Read the model definition and answer for the solid it produces. Units are mm, in the model's axes. Give positions to 0.01 mm unless a question says otherwise; leave off trailing zeros. Order: outer loops, then holes, each group sorted by start corner. A loop starts at its lowest first (then second) coordinate and runs counter-clockwise, first axis right, second up.
Item 1: Given pin 1 Ø1 at (y, z) = (-19.5, 2) entering from +X; pin 2 Ø3 at (y, z) = (-12, 17.5) entering from +X; pin 3 Ø8 at (y, z) = (-12.5, 17.5) entering from +X, each flat-ended and moving along its own axis, determine where each tip first touches the part or whether it passes through.
Item 2: A cutting plane is placed at B-B (z = -3.5). Write down the section's boundary in (x, y).
Item 3: Find the intervals of material crossed by line 1 along X through (y, z) = (4.5, -1.5); line 2 along X through (y, z) = (-9, 6.5); line 3 along Y through (x, z) = (1000, -14), in increasing order.
Item 4: A cutting plane is placed at A-A (x = 0). Write down the section's boundary in (y, z).
Item 5: The mould has two halves that part along X. Classify faces 1 (the face through (15, 23, 25)), 2 (the face through (23.846, 7.509, 0.35)), 3 (the face through (1049.988, 1.099, 0.35)), 4 (the face through (-1049.988, -1.099, 0.35)): +X half, -X half, draft (parallel to the pull), parting line (faces both ways), or undercut.
from build123d import *

# Parameters (mm, degrees)
BOSS_EXTRUDE1_DEPTH     = 25
SKETCH2_R               = 15
CUT_EXTRUDE1_DEPTH      = 51
SKETCH3_R               = 25
CUT_EXTRUDE2_DEPTH      = 26
CUT_EXTRUDE2_DEPTH_BACK = 26


with BuildPart() as part:
    # Sketch1 → Boss-Extrude1 (new body, symmetric)
    with BuildSketch(Plane.XY):
        with BuildLine():
            Line((-1000, 50), (1000, 50))
            ThreePointArc((1000, 50), (1050, 0), (1000, -50))
            Line((1000, -50), (-1000, -50))
            ThreePointArc((-1000, -50), (-1050, 0), (-1000, 50))
        make_face()
    extrude(amount=BOSS_EXTRUDE1_DEPTH, both=True)

    # Sketch2 → Cut-Extrude1 (cut, through all)
    with BuildSketch(Plane.XY.offset(25)):
        with Locations((-1000, 0)):
            Circle(SKETCH2_R)
        with Locations((1000, 0)):
            Circle(SKETCH2_R)
    extrude(amount=-CUT_EXTRUDE1_DEPTH, mode=Mode.SUBTRACT)

    # Sketch3 → Cut-Extrude2 (cut, two sides)
    with BuildSketch(Plane.XY) as cut_extrude2_sk:
        Circle(SKETCH3_R)
    extrude(amount=CUT_EXTRUDE2_DEPTH, mode=Mode.SUBTRACT)
    extrude(cut_extrude2_sk.sketch, amount=-CUT_EXTRUDE2_DEPTH_BACK, mode=Mode.SUBTRACT)


solid = part.part
Response values:
1. pin 1: stops at x = 1046.25
1. pin 2: stops at x = 1048.89
1. pin 3: stops at x = 1049.27
2. outline: (-1000, -50) - (1000, -50) arc R50 ccw to (1000, 50) - (-1000, 50) arc R50 ccw to start; hole circle Ø30 at (-1000, 0); hole circle Ø50 at (0, 0); hole circle Ø30 at (1000, 0)
3. line 1: x = -1049.8 to -1014.31, -985.69 to -24.59, 24.59 to 985.69, 1014.31 to 1049.8
3. line 2: x = -1049.18 to -1012, -988 to -23.32, 23.32 to 988, 1012 to 1049.18
3. line 3: y = -50 to -15, 15 to 50
4. outline: (-50, -25) - (-25, -25) - (-25, 25) - (-50, 25) - close; (25, -25) - (50, -25) - (50, 25) - (25, 25) - close
5. face 1: draft
5. face 2: undercut
5. face 3: +X half
5. face 4: -X half
